The listing builds one solid part. Answer for the finished solid, in the listing's coordinates (mm). Coordinates: 2 decimals unless noted, no trailing zeros. Write each question's results on one line, items separated by ' | '. Start each with the question number.
(1) Consider line 1 (Z direction, x = -59, y = 556); line 2 (Y direction, x = -23.5, z = 25.5); line 3 (Y direction, x = -32, z = -69). Determine where each line is inside the solid, lowest interval first. Write a range as from..to.
(2) Find section A-A on y = 619. State how many separate pieces and enclosed holes the cut face has, then the cut area to 3 significant figures.
(3) Given pin 1 Ø20 at (x, y) = (42, 377.5) entering from +Z; pin 2 Ø22 at (x, y) = (59, 449.5) entering from +Z; pin 3 Ø19.5 at (x, y) = (-38, 300) entering from +Z, each flat-ended and moving along its own axis, determine where each tip first touches the part or whether it passes through.
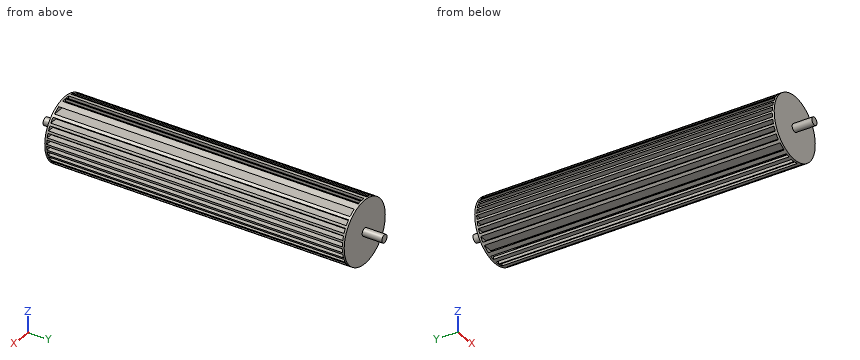
from build123d import *

# Parameters (mm, degrees)
SKETCH_1_R          = 80
EXTRUDE_1_DEPTH     = 760
CUT_EXTRUDE_START   = -5
SKETCH_2_R          = 65
CUT_EXTRUDE_1_DEPTH = 750
SKETCH_4_W          = 10
SKETCH_4_H          = 750
SKETCH_4_H_2        = 750.817396449
CUT_EXTRUDE_5_DEPTH = 781.768851838
SKETCH_5_W          = 10
SKETCH_5_H          = 750
SKETCH_5_H_2        = 749.429411824
CUT_EXTRUDE_6_DEPTH = 1100
SKETCH_6_R          = 10
EXTRUDE_2_DEPTH     = 50
EXTRUDE_START       = 50
SKETCH_7_R          = 10
EXTRUDE_3_DEPTH     = 50


with BuildPart() as part:
    # 草图1 → 凸台-拉伸1 (new body)
    with BuildSketch(Plane(origin=(0, 0, 0), x_dir=(1, 0, 0), z_dir=(0, 1, 0))):
        with Locations(Location((0, 0, 0), (0, 0, 270))):
            Circle(SKETCH_1_R)
    extrude(amount=EXTRUDE_1_DEPTH)

    # 草图2 → 切除-拉伸1 (cut)
    with BuildSketch(Plane(origin=(0, 760, 0), x_dir=(1, 0, 0), z_dir=(0, 1, 0)).offset(CUT_EXTRUDE_START)):
        with Locations(Location((0, 0, 0), (0, 0, 270))):
            Circle(SKETCH_2_R)
    extrude(amount=-CUT_EXTRUDE_1_DEPTH, mode=Mode.SUBTRACT)

    # 草图4 → 切除-拉伸5 (cut, through all)
    with BuildSketch(Plane(origin=(80, 0, 0), x_dir=(0, 0, -1), z_dir=(1, 0, 0))):
        with Locations((-67.815389673, 380)):
            Rectangle(SKETCH_4_W, SKETCH_4_H)
        with Locations((-52.815389673, 380)):
            Rectangle(SKETCH_4_W, SKETCH_4_H)
        with Locations((-37.815389673, 380)):
            Rectangle(SKETCH_4_W, SKETCH_4_H)
        with Locations((-7.815389673, 380)):
            Rectangle(SKETCH_4_W, SKETCH_4_H)
        with Locations((22.184610327, 380)):
            Rectangle(SKETCH_4_W, SKETCH_4_H)
        with Locations((52.184610327, 380)):
            Rectangle(SKETCH_4_W, SKETCH_4_H)
        with Locations((7.184610327, 380)):
            Rectangle(SKETCH_4_W, SKETCH_4_H)
        with Locations((37.184610327, 380)):
            Rectangle(SKETCH_4_W, SKETCH_4_H)
        with Locations((-22.815389673, 380)):
            Rectangle(SKETCH_4_W, SKETCH_4_H)
        with Locations((67.184610327, 379.591301776)):
            Rectangle(SKETCH_4_W, SKETCH_4_H_2)
    extrude(amount=-CUT_EXTRUDE_5_DEPTH, mode=Mode.SUBTRACT)

    # 草图5 → 切除-拉伸6 (cut)
    with BuildSketch(Plane.XY.offset(192.352939281)):
        with Locations((-19.871967952, 380)):
            Rectangle(SKETCH_5_W, SKETCH_5_H)
        with Locations((0.239093499, 380.285294088)):
            Rectangle(SKETCH_5_W, SKETCH_5_H_2)
        with Locations((12.740250466, 380)):
            Rectangle(SKETCH_5_W, SKETCH_5_H)
    extrude(amount=-CUT_EXTRUDE_6_DEPTH, mode=Mode.SUBTRACT)

    # 草图6 → 凸台-拉伸2 (add)
    with BuildSketch(Plane(origin=(0, 760, 0), x_dir=(1, 0, 0), z_dir=(0, 1, 0))):
        with Locations(Location((0, 0, 0), (0, 0, 270))):
            Circle(SKETCH_6_R)
    extrude(amount=EXTRUDE_2_DEPTH)

    # 草图7 → 凸台-拉伸3 (add)
    with BuildSketch(Plane.XZ.offset(EXTRUDE_START)):
        with Locations(Location((0, 0, 0), (0, 0, 90))):
            Circle(SKETCH_7_R)
    extrude(amount=-EXTRUDE_3_DEPTH)


solid = part.part
Values:
1) line 1: z = -47.18..-42.18, -32.18..-27.28, 27.82..32.82, 42.82..47.82 | line 2: y = 0..5, 755..760 | line 3: y = 0..4.18, 755..760
2) separate pieces: 26 | enclosed holes: 0 | area: 2,030 mm²
3) pin 1: stops at z = 73.32 | pin 2: stops at z = 62.82 | pin 3: stops at z = 74.85
